Design review of the part built by this model. Coordinates are the model's own, in mm. A direction names the side the tool comes from. Give positions to 0.01 mm unless a question says otherwise; leave off trailing zeros. Order: outer loops, then holes, each group sorted by start corner. A loop starts at its lowest first (then second) coordinate and runs counter-clockwise, first axis right, second up.
```python
from build123d import *

# Parameters (mm, degrees)
SKETCH1_R                       = 5.5
SKETCH1_R_2                     = 2.5
SKETCH1_R_3                     = 2.6
BOSS_EXTRUDE1_DEPTH             = 6
SKETCH1_3_R                     = 5.5
CUT_EXTRUDE1_DEPTH              = 6
SKETCH2_R                       = 3.25
CUT_EXTRUDE2_DEPTH              = 6
CUT_EXTRUDE3_START              = -4.5
SKETCH1_4_R                     = 5.5
CUT_EXTRUDE3_DEPTH              = 4.5
F_6_0_2361_DIAMETER_HOLE1_D     = 5.99694
F_6_0_2361_DIAMETER_HOLE1_DEPTH = 2.69833746
F_6_0_2361_DIAMETER_HOLE1_TIP   = 1.80166254
F_6_0_2361_DIAMETER_HOLE4_D     = 5.99694
F_6_0_2361_DIAMETER_HOLE4_DEPTH = 4.19833746
F_6_0_2361_DIAMETER_HOLE4_TIP   = 1.80166254
SKETCH9_R                       = 4
CUT_EXTRUDE4_DEPTH              = 15
F_6_0_2361_DIAMETER_HOLE3_D     = 5.99694
F_6_0_2361_DIAMETER_HOLE3_DEPTH = 73
F_6_0_2361_DIAMETER_HOLE3_TIP   = 1.80166254
CHAMFER1_SIZE                   = 0.5
CHAMFER2_SIZE                   = 0.5


with BuildPart() as part:
    # Sketch1 → Boss-Extrude1 (new, symmetric)
    # profile 1 of 4: a face of its own
    with BuildSketch(Plane(origin=(0, 0, 0), x_dir=(1, 0, 0), z_dir=(0, 1, 0))):
        with BuildLine():
            ThreePointArc((58, 40), (66.485281374, 36.485281374), (70, 28))
            Line((70, 28), (70, -28))
            ThreePointArc((70, -28), (66.485281374, -36.485281374), (58, -40))
            Line((58, -40), (-58, -40))
            Line((-58, -40), (-70, -28))
            Line((-70, -28), (-70, 28))
            Line((-70, 28), (-58, 40))
            Line((-58, 40), (58, 40))
        make_face()
        with Locations((-35, -15)):
            Circle(SKETCH1_R, mode=Mode.SUBTRACT)
        with Locations((-35, 25)):
            Circle(SKETCH1_R, mode=Mode.SUBTRACT)
        with Locations((-35, 5)):
            Circle(SKETCH1_R, mode=Mode.SUBTRACT)
        with Locations(Location((-3, -3.5, 0), (0, 0, 270))):
            Circle(SKETCH1_R_2, mode=Mode.SUBTRACT)
        with Locations(Location((22, -28.5, 0), (0, 0, 270))):
            Circle(SKETCH1_R_2, mode=Mode.SUBTRACT)
        with Locations(Location((47, -3.5, 0), (0, 0, 270))):
            Circle(SKETCH1_R_2, mode=Mode.SUBTRACT)
        with Locations(Location((22, 21.5, 0), (0, 0, 270))):
            Circle(SKETCH1_R_2, mode=Mode.SUBTRACT)
        with Locations(Location((60, -30, 0), (0, 0, 270))):
            Circle(SKETCH1_R_3, mode=Mode.SUBTRACT)
        with Locations(Location((60, 30, 0), (0, 0, 270))):
            Circle(SKETCH1_R_3, mode=Mode.SUBTRACT)
        with Locations(Location((-60, -30, 0), (0, 0, 270))):
            Circle(SKETCH1_R_3, mode=Mode.SUBTRACT)
        with Locations(Location((-60, 30, 0), (0, 0, 270))):
            Circle(SKETCH1_R_3, mode=Mode.SUBTRACT)
        with Locations(Location((-35, 15, 0), (0, 0, 270))):
            Circle(SKETCH1_R_2, mode=Mode.SUBTRACT)
        with Locations(Location((-35, -5, 0), (0, 0, 270))):
            Circle(SKETCH1_R_2, mode=Mode.SUBTRACT)
    # profile 2 of 4: a face of its own
    with BuildSketch(Plane(origin=(0, 0, 0), x_dir=(1, 0, 0), z_dir=(0, 1, 0))):
        with Locations((-35, -15)):
            Circle(SKETCH1_R)
    # profile 3 of 4: a face of its own
    with BuildSketch(Plane(origin=(0, 0, 0), x_dir=(1, 0, 0), z_dir=(0, 1, 0))):
        with Locations((-35, 5)):
            Circle(SKETCH1_R)
    # profile 4 of 4: a face of its own
    with BuildSketch(Plane(origin=(0, 0, 0), x_dir=(1, 0, 0), z_dir=(0, 1, 0))):
        with Locations((-35, 25)):
            Circle(SKETCH1_R)
    extrude(amount=BOSS_EXTRUDE1_DEPTH, both=True)

    # Sketch1_3 → Cut-Extrude1 (cut)
    with BuildSketch(Plane(origin=(0, 0, 0), x_dir=(1, 0, 0), z_dir=(0, 1, 0))):
        with Locations(Location((-35, 25, 0), (0, 0, 270))):
            Circle(SKETCH1_3_R)
        with Locations(Location((-35, -15, 0), (0, 0, 270))):
            Circle(SKETCH1_3_R)
    extrude(amount=CUT_EXTRUDE1_DEPTH, mode=Mode.SUBTRACT)

    # Sketch2 → Cut-Extrude2 (cut)
    with BuildSketch(Plane(origin=(0, 0, 0), x_dir=(1, 0, 0), z_dir=(0, 1, 0))):
        with Locations(Location((-35, 25, 0), (0, 0, 270))):
            Circle(SKETCH2_R)
        with Locations(Location((-35, -15, 0), (0, 0, 90))):
            Circle(SKETCH2_R)
    extrude(amount=-CUT_EXTRUDE2_DEPTH, mode=Mode.SUBTRACT)

    # Sketch1_4 → Cut-Extrude3 (cut)
    with BuildSketch(Plane(origin=(0, 0, 0), x_dir=(1, 0, 0), z_dir=(0, 1, 0)).offset(CUT_EXTRUDE3_START)):
        with Locations(Location((-35, 5, 0), (0, 0, 270))):
            Circle(SKETCH1_4_R)
    extrude(amount=-CUT_EXTRUDE3_DEPTH, mode=Mode.SUBTRACT)

    # 6 _0.2361_ Diameter Hole1
    with Locations(Plane(origin=(0, -4.5, 0), x_dir=(-1, 0, 0), z_dir=(0, -1, 0))):
        with Locations((35, 5)):
            Hole(F_6_0_2361_DIAMETER_HOLE1_D / 2, depth=F_6_0_2361_DIAMETER_HOLE1_DEPTH)
            with Locations((0, 0, -(F_6_0_2361_DIAMETER_HOLE1_DEPTH + F_6_0_2361_DIAMETER_HOLE1_TIP / 2))):  # 118° drill point
                Cone(0, F_6_0_2361_DIAMETER_HOLE1_D / 2, F_6_0_2361_DIAMETER_HOLE1_TIP, mode=Mode.SUBTRACT)

    # 6 _0.2361_ Diameter Hole4
    with Locations(Plane(origin=(0, -6, 0), x_dir=(-1, 0, 0), z_dir=(0, -1, 0))):
        with Locations((-14, 5)):
            Hole(F_6_0_2361_DIAMETER_HOLE4_D / 2, depth=F_6_0_2361_DIAMETER_HOLE4_DEPTH)
            with Locations((0, 0, -(F_6_0_2361_DIAMETER_HOLE4_DEPTH + F_6_0_2361_DIAMETER_HOLE4_TIP / 2))):  # 118° drill point
                Cone(0, F_6_0_2361_DIAMETER_HOLE4_D / 2, F_6_0_2361_DIAMETER_HOLE4_TIP, mode=Mode.SUBTRACT)

    # Sketch9 → Cut-Extrude4 (cut)
    with BuildSketch(Plane.ZY.offset(70)):
        with Locations((-5, 0)):
            Circle(SKETCH9_R)
    extrude(amount=-CUT_EXTRUDE4_DEPTH, mode=Mode.SUBTRACT)

    # 6 _0.2361_ Diameter Hole3
    with Locations(Plane.ZY.offset(55)):
        with Locations((-5, 0)):
            Hole(F_6_0_2361_DIAMETER_HOLE3_D / 2, depth=F_6_0_2361_DIAMETER_HOLE3_DEPTH)
            with Locations((0, 0, -(F_6_0_2361_DIAMETER_HOLE3_DEPTH + F_6_0_2361_DIAMETER_HOLE3_TIP / 2))):  # 118° drill point
                Cone(0, F_6_0_2361_DIAMETER_HOLE3_D / 2, F_6_0_2361_DIAMETER_HOLE3_TIP, mode=Mode.SUBTRACT)

    # Chamfer1
    chamfer1_edges = [part.edges().sort_by_distance(p)[0] for p in [
        (-35, 6, 2.5),
        (-3, 6, 1),
        (22, 6, 26),
        (47, 6, 1),
        (22, 6, -24),
        (60, 6, 27.4),
        (60, 6, -32.6),
        (66.485281374, 6, -36.485281374),
        (0, 6, -40),
        (-64, 6, -34),
        (-35, 6, -30.5),
        (-35, 6, 9.5),
        (-70, 6, 0),
        (-64, 6, 34),
        (0, 6, 40),
        (66.485281374, 6, 36.485281374),
        (70, 6, 0),
        (-60, 6, 27.4),
        (-60, 6, -32.6),
        (-35, 6, -17.5),
    ]]
    chamfer(chamfer1_edges, length=CHAMFER1_SIZE)

    # Chamfer2
    chamfer2_edges = [part.edges().sort_by_distance(p)[0] for p in [
        (-35, -6, 2.5),
        (-35, -6, -17.5),
        (-60, -6, -32.6),
        (-60, -6, 27.4),
        (70, -6, 0),
        (66.485281374, -6, 36.485281374),
        (0, -6, 40),
        (-64, -6, 34),
        (-70, -6, 0),
        (-64, -6, -34),
        (0, -6, -40),
        (66.485281374, -6, -36.485281374),
        (60, -6, -32.6),
        (60, -6, 27.4),
        (22, -6, -24),
        (47, -6, 1),
        (22, -6, 26),
        (-3, -6, 1),
        (-35, -6, -28.25),
        (-35, -6, 18.25),
        (-35, -6, -10.5),
        (11.00153, -6, -5),
    ]]
    chamfer(chamfer2_edges, length=CHAMFER2_SIZE)


solid = part.part
```
1. Take a section at A-A (z = -15). State the section outline as (x, y) points.
Recorded:
outline: (-70, -5.5) - (-69.5, -6) - (-38, -6) - (-37.5, -5.5) - (-37.5, 5.5) - (-38, 6) - (-69.5, 6) - (-70, 5.5) - close; (-32.5, -5.5) - (-32, -6) - (69.5, -6) - (70, -5.5) - (70, 5.5) - (69.5, 6) - (-32, 6) - (-32.5, 5.5) - close
2. Take a section at B-B (x = 4). State the section outline as (y, z) points, then the cut area to 3 significant figures.
Recorded:
outline: (-6, -39.5) - (-5.5, -40) - (5.5, -40) - (6, -39.5) - (6, 39.5) - (5.5, 40) - (-5.5, 40) - (-6, 39.5) - close; hole circle Ø6 at (0, -5)
area: 931 mm2
3. Machinability: for faces 1 (the face through (13.35, -3.625, -2.073)), 2 (the face through (-1, 0, -40)), 3 (the face through (-18, 3, -5)), which of the approach directions +Z, -Z, +X, -X, +Y, -Y give a long, thin tool a straight path to every point of the face, cutting with its end or side? Answer none if there is none.
Recorded:
face 1: -Y
face 2: -Z, +X, -X, +Y, -Y
face 3: -X
4. Draft analysis for pull direction Z (two halves, no side actions). For faces 4 (the face through (-1, -6, -1)), 5 (the face through (-63.74, -5.75, 33.91)), 6 (the face through (-35, 0, 19)), state which applies: pulls with the +Z half, pulls with the -Z half, needs draft (parallel to the pull), parting line crosses it, or undercut.
Recorded:
face 4: needs draft
face 5: pulls with the +Z half
face 6: undercut
5. For pin 1 (5 mm diameter, centred on x = -35, z = -5, fed in from -Y); pin 2 (3 mm diameter, centred on x = -3, z = 3.5, fed in from -Y); pin 3 (3.5 mm diameter, centred on y = 0, z = -5, fed in from -X), all flat-tipped, find the tip position at first contact; note any pin that passes through.
Recorded:
pin 1: stops at y = 1.66
pin 2: passes through
pin 3: stops at x = 18.75
6. For line 1 along X through (y, z) = (-4.75, -5); line 2 along X through (y, z) = (-4.75, -22); line 3 along X through (y, z) = (-4.4, 30), list the stretches that pass through material, from the lowest coordinate up.
Recorded:
line 1: x = -70 to -40.5, -29.5 to 11, 17 to 70
line 2: x = -70 to -36.25, -33.75 to 19.55, 24.45 to 70
line 3: x = -68 to -62.6, -57.4 to 20, 24 to 57.4, 62.6 to 69.83
7. Take a section at C-C (x = -35). State how many separate pieces and enclosed holes the cut face has, then the cut area to 3 significant figures.
Recorded:
separate pieces: 5
enclosed holes: 0
area: 570 mm2
